from build123d import *

# Parameters (mm, degrees)
SKETCH1_W           = 71.28
SKETCH1_H           = 42.64
BOSS_EXTRUDE1_DEPTH = 6.35
SKETCH3_W           = 12.7
SKETCH3_H           = 42.64
BOSS_EXTRUDE3_DEPTH = 12.7
SKETCH4_W           = 12.7
SKETCH4_H           = 12.7
BOSS_EXTRUDE4_DEPTH = 27.94
SKETCH6_W           = 12.7
SKETCH6_H           = 12.676175504
BOSS_EXTRUDE5_DEPTH = 27.94
SKETCH7_R           = 2.286
SKETCH7_R_2         = 2.285
CUT_EXTRUDE1_DEPTH  = 63.267019151
SKETCH10_W          = 16.129
SKETCH10_H          = 71.046005576
BOSS_EXTRUDE6_DEPTH = 6.35
SKETCH11_R          = 2.413
CUT_EXTRUDE2_DEPTH  = 6.35
CHAMFER1_SIZE       = 2.38
FILLET1_R           = 2.38


with BuildPart() as part:
    # Sketch1 → Boss-Extrude1 (new body)
    with BuildSketch(Plane(origin=(0, 0, 0), x_dir=(1, 0, 0), z_dir=(0, 1, 0))):
        with Locations((-1.22975773, -8.11115762)):
            Rectangle(SKETCH1_W, SKETCH1_H)
    extrude(amount=BOSS_EXTRUDE1_DEPTH)

    # Sketch3 → Boss-Extrude3 (add)
    with BuildSketch(Plane(origin=(0, 6.35, 0), x_dir=(1, 0, 0), z_dir=(0, 1, 0))):
        with Locations((-30.51975773, -8.11115762)):
            Rectangle(SKETCH3_W, SKETCH3_H)
    extrude(amount=BOSS_EXTRUDE3_DEPTH)

    # Sketch4 → Boss-Extrude4 (add)
    with BuildSketch(Plane(origin=(0, 19.05, 0), x_dir=(1, 0, 0), z_dir=(0, 1, 0))):
        with Locations((-30.51975773, -23.08115762)):
            Rectangle(SKETCH4_W, SKETCH4_H)
    extrude(amount=BOSS_EXTRUDE4_DEPTH)

    # Sketch6 → Boss-Extrude5 (add)
    with BuildSketch(Plane(origin=(0, 19.05, 0), x_dir=(1, 0, 0), z_dir=(0, 1, 0))):
        with Locations((-30.51975773, 6.870754628)):
            Rectangle(SKETCH6_W, SKETCH6_H)
    extrude(amount=BOSS_EXTRUDE5_DEPTH)

    # Sketch7 → Cut-Extrude1 (cut, through all)
    with BuildSketch(Plane(origin=(0, 6.35, 0), x_dir=(1, 0, 0), z_dir=(0, 1, 0))):
        with Locations(Location((6.23024227, -8.11115762, 0), (0, 0, 270))):
            Circle(SKETCH7_R)
        with Locations(Location((31.63024227, -8.11115762, 0), (0, 0, 270))):
            Circle(SKETCH7_R)
        with Locations(Location((12.73024227, 4.08884238, 0), (0, 0, 270))):
            Circle(SKETCH7_R_2)
        with Locations(Location((12.83024227, -20.31115762, 0), (0, 0, 270))):
            Circle(SKETCH7_R_2)
        with Locations(Location((26.63024227, 4.08884238, 0), (0, 0, 270))):
            Circle(SKETCH7_R_2)
        with Locations(Location((26.73024227, -20.31115762, 0), (0, 0, 270))):
            Circle(SKETCH7_R_2)
    extrude(amount=-CUT_EXTRUDE1_DEPTH, mode=Mode.SUBTRACT)

    # Sketch10 → Boss-Extrude6 (add)
    with BuildSketch(Plane(origin=(0, 6.35, 0), x_dir=(1, 0, 0), z_dir=(0, 1, 0))):
        with Locations((42.47474227, -8.11115762)):
            Rectangle(SKETCH10_W, SKETCH10_H)
    extrude(amount=-BOSS_EXTRUDE6_DEPTH)

    # Sketch11 → Cut-Extrude2 (cut)
    with BuildSketch(Plane(origin=(0, 6.35, 0), x_dir=(1, 0, 0), z_dir=(0, 1, 0))):
        with Locations(Location((42.41124227, 21.061845168, 0), (0, 0, 270))):
            Circle(SKETCH11_R)
        with Locations(Location((42.41124227, -37.284160408, 0), (0, 0, 270))):
            Circle(SKETCH11_R)
    extrude(amount=-CUT_EXTRUDE2_DEPTH, mode=Mode.SUBTRACT)

    # Chamfer1
    chamfer1_edges = [part.edges().sort_by_distance(p)[0] for p in [
        (-1.22975773, 0, 29.43115762),
        (-36.86975773, 0, 8.11115762),
        (-1.22975773, 0, -13.20884238),
        (34.41024227, 0, -20.310343774),
        (34.41024227, 0, 36.532659014),
        (42.47474227, 0, -27.411845168),
        (50.53924227, 0, 8.11115762),
        (42.47474227, 0, 43.634160408),
    ]]
    chamfer(chamfer1_edges, length=CHAMFER1_SIZE)

    # Fillet1
    fillet1_edges = [part.edges().sort_by_distance(p)[0] for p in [
        (5.12024227, 6.35, 29.43115762),
        (-24.16975773, 6.35, 8.11115762),
        (-24.16975773, 26.67, 29.43115762),
        (-24.16975773, 26.67, -13.20884238),
        (-24.16975773, 33.02, 16.73115762),
        (-36.86975773, 33.02, 16.73115762),
        (-36.86975773, 33.02, -0.532666876),
        (-24.16975773, 33.02, -0.532666876),
        (5.12024227, 6.35, -13.20884238),
        (-36.86975773, 24.685, 29.43115762),
        (-36.86975773, 24.685, -13.20884238),
        (34.41024227, 6.35, -20.310343774),
        (34.41024227, 6.35, 36.532659014),
        (42.47474227, 6.35, 43.634160408),
        (50.53924227, 6.35, 8.11115762),
        (42.47474227, 6.35, -27.411845168),
    ]]
    fillet(fillet1_edges, radius=FILLET1_R)


solid = part.part
Model file for the job. Use its own axes, mm. A direction names the side the tool comes from. Give positions to 0.01 mm unless a question says otherwise; leave off trailing zeros. Loops run counter-clockwise (first coordinate to the right, second up) from the corner with the lowest first, then second, coordinate; pieces in that order, holes last.
Item 1: Mould opens along Z. For faces 6 (the face through (-31, 33, -0.533)), 7 (the face through (-24.17, 15, 8)), 8 (the face through (-31, 19.05, 8)), 9 (the face through (42.59, 5.67, 42.92)) say: +Z half, -Z half, draft (parallel to the pull), parting line (faces both ways), or undercut.
Check values:
face 6: undercut
face 7: draft
face 8: undercut
face 9: +Z half
Item 2: Slice it at A-A (y = 28.5). Write the cut outline in (x, z).
Check values:
outline: (-36.87, -10.83) arc R2.38 ccw to (-34.49, -13.21) - (-26.55, -13.21) arc R2.38 ccw to (-24.17, -10.83) - (-24.17, -2.91) arc R2.38 ccw to (-26.55, -0.53) - (-34.49, -0.53) arc R2.38 ccw to (-36.87, -2.91) - close; (-36.87, 19.11) arc R2.38 ccw to (-34.49, 16.73) - (-26.55, 16.73) arc R2.38 ccw to (-24.17, 19.11) - (-24.17, 27.05) arc R2.38 ccw to (-26.55, 29.43) - (-34.49, 29.43) arc R2.38 ccw to (-36.87, 27.05) - close
Item 3: Which spindle directions (+Z, -Z, +X, -X, +Y, -Y) get a long thin tool onto all of the face, cutting with end or side? Do faces 1 (the face through (-24.848, 33.216, 17.447)), 2 (the face through (-28, 20, 29.431)), 3 (the face through (-28, 20, -13.209)), 4 (the face through (7.91, 5.671, -12.493)), 5 (the face through (-0.2, 1.21, -12.04)). Say none if no direction does.
Check values:
face 1: +X, +Y
face 2: +Z, -X, +Y, -Y
face 3: -Z, -X, +Y, -Y
face 4: -Z, +Y
face 5: -Z, -X, -Y
Item 4: Drop flat-ended pins along their axis: P1, Ø6.5, axis at x = -32.5, z = 4, coming from the +Y side; P2, Ø3.5, axis at x = 6.23, z = 8.11, coming from the -Y side; P3, Ø8, axis at y = 35.5, z = -7, coming from the +X side; P4, Ø5, axis at x = -6.5, z = -14.5, coming from the +Y side. Give the stop position or say it passes through.
Check values:
P1: stops at y = 19.05
P2: passes through
P3: stops at x = -24.17
P4: stops at y = 6.04
Item 5: Slice it at B-B (z = 25.5). Write the cut outline in (x, y), plus the area to 3 significant figures.
Check values:
outline: (-36.87, 2.38) - (-34.49, 0) - (48.16, 0) - (50.54, 2.38) - (50.54, 3.97) arc R2.38 ccw to (48.16, 6.35) - (-21.79, 6.35) arc R2.38 cw to (-24.17, 8.73) - (-24.17, 46.99) - (-36.87, 46.99) - close
area: 1,070 mm2
Item 6: Slice it at D-D (z = 7). Write the cut outline in (x, y), plus the area to 3 significant figures.
Check values:
outline: (-36.87, 2.38) - (-34.49, 0) - (4.23, 0) - (4.23, 6.35) - (-21.79, 6.35) arc R2.38 cw to (-24.17, 8.73) - (-24.17, 19.05) - (-36.87, 19.05) - close; (8.23, 0) - (29.63, 0) - (29.63, 6.35) - (8.23, 6.35) - close; (33.63, 0) - (48.16, 0) - (50.54, 2.38) - (50.54, 3.97) arc R2.38 ccw to (48.16, 6.35) - (33.63, 6.35) - close
area: 660 mm2
Item 7: Drill centre lines: line 1 along Z through (x, y) = (-31, 39.5); line 2 along Y through (x, z) = (-15, -5); line 3 along Z through (x, y) = (-25, 23.5). Where is each one in solid material? Low to high.
Check values:
line 1: z = -13.21 to -0.53, 16.73 to 29.43
line 2: y = 0 to 6.35
line 3: z = -12.64 to -1.11, 17.3 to 28.86
Item 8: Slice it at C-C (x = -4). Write the cut outline in (y, z).
Check values:
outline: (0, -10.83) - (2.38, -13.21) - (3.97, -13.21) arc R2.38 ccw to (6.35, -10.83) - (6.35, 27.05) arc R2.38 ccw to (3.97, 29.43) - (2.38, 29.43) - (0, 27.05) - close
